Autodesk Inventor part; units mm, degrees
ref_plane "YZ Plane" through (0, 0, 0) normal (1, 0, 0) x (0, 1, 0)
ref_plane "XZ Plane" through (0, 0, 0) normal (0, 1, 0) x (-1, 0, 0)
ref_plane "XY Plane" through (0, 0, 0) normal (0, 0, 1) x (1, 0, 0)
sketch "Sketch1" plane through (0, 0, 0) normal (0, 0, 1) x (1, 0, 0)
  line L0 (-30, -30) -> (30, -30)
  line L1 (30, -30) -> (30, 30)
  line L2 (30, 30) -> (-30, 30)
  line L3 (-30, 30) -> (-30, -30)
  line L4 (-30, -30) -> (30, 30) construction
  line L5 (30, -30) -> (-30, 30) construction
  line L6 (15.1, -15.1) -> (-15.1, -15.1)
  line L7 (-15.1, -15.1) -> (-15.1, 15.1)
  line L8 (-15.1, 15.1) -> (15.1, 15.1)
  line L9 (15.1, 15.1) -> (15.1, -15.1)
  line L10 (15.1, -15.1) -> (-15.1, 15.1) construction
  line L11 (-15.1, -15.1) -> (15.1, 15.1) construction
  circle A0 centre (-23, -23) radius 2.75
  circle A1 centre (23, -23) radius 2.75
  circle A2 centre (23, 23) radius 2.75
  circle A3 centre (-23, 23) radius 2.75
  line L12 (25.75, 25.75) -> (-25.75, 25.75) construction
  line L13 (-25.75, 25.75) -> (-25.75, -25.75) construction
  line L14 (-25.75, -25.75) -> (25.75, -25.75) construction
  line L15 (25.75, -25.75) -> (25.75, 25.75) construction
  line L16 (25.75, 25.75) -> (-25.75, -25.75) construction
  line L17 (-25.75, 25.75) -> (25.75, -25.75) construction
  line L18 (23, 23) -> (-23, 23) construction
  line L19 (-23, 23) -> (-23, -23) construction
  line L20 (-23, -23) -> (23, -23) construction
  line L21 (23, -23) -> (23, 23) construction
  line L22 (23, 23) -> (-23, -23) construction
  line L23 (-23, 23) -> (23, -23) construction
  point P0 (0, 0)
  dimension "d172" = 30.2
  dimension "d190" = 5.5
  dimension "d191" = 46
  dimension "d192" = 60
extrude "Plate5" add sketch "Sketch1" along normal blind 3
fillet "Corner Round1" radius 2 4 edges at (30, 30, 1.5) (-30, 30, 1.5) (-30, -30, 1.5) (30, -30, 1.5)
fillet "Corner Round2" radius 0.5 4 edges at (-15.1, 15.1, 1.5) (-15.1, -15.1, 1.5) (15.1, -15.1, 1.5) (15.1, 15.1, 1.5)
properties part number "PRS 1425 DrSysB Way FLANGE_1200" material "Stainless Steel"
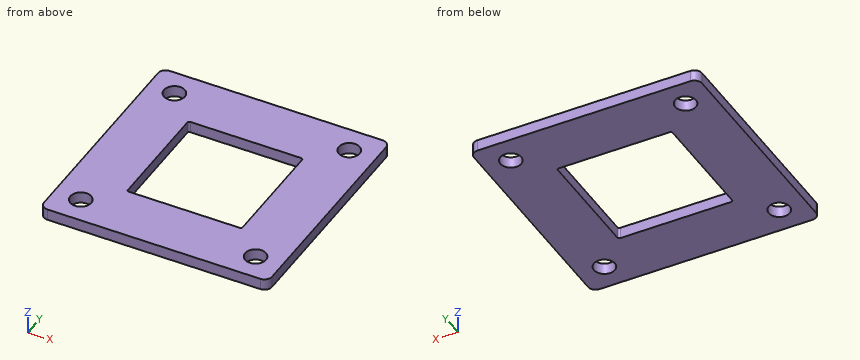
Source: CAD feature listing. Evaluate the final solid. Frame: model axes, mm. Coordinates: 2 decimals unless noted, no trailing zeros. Loops run counter-clockwise (first coordinate to the right, second up) from the corner with the lowest first, then second, coordinate; pieces in that order, holes last. Notation, with made-up numbers: (53, -27.75) - (76, -27.75) arc R31 cw to (76, 8.25) - close; hole circle Ø5 at (-32, 20.5). An arc over 180 degrees is marked (long way). Return JSON: item names as keys, results as strings.
Q1. Section A-A, the plane x = 6.5. Return loops of the section in (y, z).
Results:
{"outline": "(-30, 0) - (-15.1, 0) - (-15.1, 3) - (-30, 3) - close; (15.1, 0) - (30, 0) - (30, 3) - (15.1, 3) - close"}
Q2. Section B-B, the plane y = -23. Return loops of the section in (x, z), plus the area to 3 significant figures.
Results:
{"outline": "(-30, 0) - (-25.75, 0) - (-25.75, 3) - (-30, 3) - close; (-20.25, 0) - (20.25, 0) - (20.25, 3) - (-20.25, 3) - close; (25.75, 0) - (30, 0) - (30, 3) - (25.75, 3) - close", "area": "147 mm2"}
Q3. Section C-C, the plane z = 0.9. Return loops of the section in (x, y).
Results:
{"outline": "(-30, -28) arc R2 ccw to (-28, -30) - (28, -30) arc R2 ccw to (30, -28) - (30, 28) arc R2 ccw to (28, 30) - (-28, 30) arc R2 ccw to (-30, 28) - close; hole circle Ø5.5 at (-23, -23); hole circle Ø5.5 at (-23, 23); hole (-15.1, -14.6) arc R0.5 ccw to (-14.6, -15.1) - (14.6, -15.1) arc R0.5 ccw to (15.1, -14.6) - (15.1, 14.6) arc R0.5 ccw to (14.6, 15.1) - (-14.6, 15.1) arc R0.5 ccw to (-15.1, 14.6) - close; hole circle Ø5.5 at (23, -23); hole circle Ø5.5 at (23, 23)"}
Q4. Material intervals for line 1 along Y through (x, z) = (9.5, 2.25); line 2 along Y through (x, z) = (23, 0.7), sorted ascending.
Results:
{"line 1": "-30 to -15.1, 15.1 to 30", "line 2": "-30 to -25.75, -20.25 to 20.25, 25.75 to 30"}
